```python
from build123d import *

# Parameters (mm, degrees)
F1_DEPTH = 5
F2_W     = 30
F2_H     = 50
F3_DEPTH = 5
F4_R     = 1.625
F5_DEPTH = 25
F6_R     = 5


with BuildPart() as f1:
    # F0 (on Top) → F1 (new body)
    with BuildSketch(Plane.XY):
        Polygon((-15, 50), (-15, 0), (0, 0), (15, 0), (15, 50), (0, 50), align=None)
        Polygon((3.07439, 18.2625), (3.07439, 14.7125), (0, 12.9375), (-3.07439, 14.7125), (-3.07439, 18.2625), (0, 20.0375), align=None, mode=Mode.SUBTRACT)
        Polygon((3.07439, 29.7125), (0, 27.9375), (-3.07439, 29.7125), (-3.07439, 33.2625), (0, 35.0375), (3.07439, 33.2625), align=None, mode=Mode.SUBTRACT)
    extrude(amount=-F1_DEPTH)

    # F2 (on Top) → F3 (join)
    with BuildSketch(Plane.XY):
        with Locations((0, 25)):
            Rectangle(F2_W, F2_H)
    extrude(amount=F3_DEPTH)

    # F4 (on face) → F5 (cut)
    with BuildSketch(Plane(origin=(0, 0, -5), x_dir=(1, 0, 0), z_dir=(0, 0, -1))):
        with Locations((0, -16.4875)):
            Circle(F4_R)
        with Locations((0, -31.4875)):
            Circle(F4_R)
    extrude(amount=-F5_DEPTH, mode=Mode.SUBTRACT)

    # F6
    f6_edges = [f1.edges().sort_by_distance(p)[0] for p in [
        (0, 0, -5),
        (-15, 25, -5),
        (15, 25, -5),
        (0, 50, -5),
        (15, 50, 0),
        (-15, 0, 0),
        (-15, 50, 0),
        (15, 0, 0),
    ]]
    fillet(f6_edges, radius=F6_R)


solid = f1.part
```
Can you work these out from the model? Positions are in its coordinate system, mm. A direction names the side the tool comes from. Coordinates: 2 decimals unless noted, no trailing zeros. Loops run counter-clockwise (first coordinate to the right, second up) from the corner with the lowest first, then second, coordinate; pieces in that order, holes last.
1) Thinking about a two-plate mould opening in Y: for faces 3 (the flat face through (15, 25, 2)), 4 (the cylindrical face through (-14, 48, 2)), 5 (the flat face through (-1, 30, 0)), which applies, pulls with the +Y half, pulls with the -Y half, needs draft (parallel to the pull), parting line crosses it, or undercut?
2) Imagine slicing it at C-C on y = 41.5. List the corners of the cut face in (x, z) for me, plus the area to 3 significant figures.
3) Imagine slicing it at B-B on x = -7.75. List the corners of the cut face in (y, z) for me, plus the area to 3 significant figures.
4) Which directions (+Z, -Z, +X, -X, +Y, -Y) give clear straight access to the entire face, cutting with the end or side of a thin tool? Please do faces 1 (the cylindrical face through (-14, 25, -3)), 2 (the flat face through (1.52, 19.16, -2.46)).
5) Imagine slicing it at A-A on z = -2.25. List the corners of the cut face in (x, y) for me, plus the area to 3 significant figures.
6) Imagine slicing it at D-D on z = 3.75. State how many separate pieces and enclosed holes the cut face has, plus the area to 3 significant figures.
7) I need wall thicknesses on probe 1 along Y at (x, z) = (0, 1.25); probe 2 along Y at (x, z) = (-1, 3.75); probe 3 along X at (y, z) = (16.5, -0.25). Which ranges of each line are inside material? Lowest first, please.
8) For pin 1 (3 mm diameter, centred on y = 16.5, z = -2, fed in from +X); pin 2 (2 mm diameter, centred on y = 25, z = -2, fed in from -X); pin 3 (3 mm diameter, centred on y = 16.5, z = -3.5, fed in from -X), each with a flat end and sliding along its axis, tell me the tip position at first contact or that it passes through.
Completed:
1. face 3: needs draft
1. face 4: pulls with the +Y half
1. face 5: undercut
2. outline: (-15, 0) arc R5 ccw to (-10, -5) - (10, -5) arc R5 ccw to (15, 0) - (15, 5) - (-15, 5) - close
2. area: 289 mm2
3. outline: (0, 0) arc R5 ccw to (5, -5) - (45, -5) arc R5 ccw to (50, 0) - (50, 5) - (0, 5) - close
3. area: 489 mm2
4. face 1: -Z, -X, +Y, -Y
4. face 2: -Z
5. outline: (-14.47, 5) arc R4.47 ccw to (-10, 0.53) - (10, 0.53) arc R4.47 ccw to (14.47, 5) - (14.47, 45) arc R4.47 ccw to (10, 49.47) - (-10, 49.47) arc R4.47 ccw to (-14.47, 45) - close; hole (-3.07, 14.71) - (0, 12.94) - (3.07, 14.71) - (3.07, 18.26) - (0, 20.04) - (-3.07, 18.26) - close; hole (-3.07, 29.71) - (0, 27.94) - (3.07, 29.71) - (3.07, 33.26) - (0, 35.04) - (-3.07, 33.26) - close
5. area: 1,330 mm2
6. separate pieces: 1
6. enclosed holes: 2
6. area: 1,460 mm2
7. probe 1: y = 0 to 14.86, 18.11 to 29.86, 33.11 to 50
7. probe 2: y = 0 to 15.21, 17.77 to 30.21, 32.77 to 50
7. probe 3: x = -14.99 to -3.07, 3.07 to 14.99
8. pin 1: stops at x = 14.97
8. pin 2: stops at x = -14.9
8. pin 3: stops at x = -14.58
